from build123d import *

# Parameters (mm, degrees)
SKETCH1_R           = 4
SKETCH1_R_2         = 1.85
BOSS_EXTRUDE1_DEPTH = 3.175


with BuildPart() as part:
    # Sketch1 → Boss-Extrude1 (new body)
    with BuildSketch(Plane.XY):
        with BuildLine():
            Line((-38.1, 100), (38.1, 100))
            Line((38.1, 100), (38.1, 0))
            ThreePointArc((38.1, 0), (0, -38.1), (-38.1, 0))
            Line((-38.1, 0), (-38.1, 100))
        make_face()
        Circle(SKETCH1_R, mode=Mode.SUBTRACT)
        with Locations((-8, 0)):
            Circle(SKETCH1_R_2, mode=Mode.SUBTRACT)
        with Locations((0, -8)):
            Circle(SKETCH1_R_2, mode=Mode.SUBTRACT)
        with Locations((0, 8)):
            Circle(SKETCH1_R_2, mode=Mode.SUBTRACT)
        with Locations((8, 0)):
            Circle(SKETCH1_R_2, mode=Mode.SUBTRACT)
    extrude(amount=BOSS_EXTRUDE1_DEPTH)


solid = part.part
Read the model definition and answer for the solid it produces. Units are mm, in the model's axes. Coordinates: 2 decimals unless noted, no trailing zeros. Loops run counter-clockwise (first coordinate to the right, second up) from the corner with the lowest first, then second, coordinate; pieces in that order, holes last.
Q1. The part is cut by section D-D on x = 16. Write down the section's boundary in (y, z) (3 decimals).
Q2. This flat-tipped pin is pushed along its axis until it touches: pin 1 Ø3 at (x, y) = (29, 57) entering from -Z. Where does it stop, or does it pass through?
Q3. Consider probe 1 along Y at (x, z) = (0, 2.1); probe 2 along Y at (x, z) = (1, 2.9); probe 3 along Y at (x, z) = (-2, 0.75). Determine where each line is inside the solid, lowest interval first.
Q4. The part is cut by section C-C on x = -8. Write down the section's boundary in (y, z) (3 decimals), and give its area (3 significant figures).
Q5. The part is cut by section B-B on z = 1.1. Write down the section's boundary in (x, y), and give its area (3 significant figures).
Q6. The part is cut by section A-A on y = 8. Write down the section's boundary in (x, z) (3 decimals), and give its area (3 significant figures).
Q7. The mould has two halves that part along Y. Classify faces 1 (the face through (38.1, 51, 2)), 2 (the face through (-0.401, 6.194, 1.565)), 3 (the face through (0.84, -38.09, 1.57)): +Y half, -Y half, draft (parallel to the pull), parting line (faces both ways), or undercut.
Results below:
1. outline: (-34.578, 0) - (100, 0) - (100, 3.175) - (-34.578, 3.175) - close
2. pin 1: stops at z = 0
3. probe 1: y = -38.1 to -9.85, -6.15 to -4, 4 to 6.15, 9.85 to 100
3. probe 2: y = -38.09 to -9.56, -6.44 to -3.87, 3.87 to 6.44, 9.56 to 100
3. probe 3: y = -38.05 to -3.46, 3.46 to 100
4. outline: (-37.251, 0) - (-1.85, 0) - (-1.85, 3.175) - (-37.251, 3.175) - close; (1.85, 0) - (100, 0) - (100, 3.175) - (1.85, 3.175) - close
4. area: 424 mm2
5. outline: (-38.1, 0) arc R38.1 ccw to (38.1, 0) - (38.1, 100) - (-38.1, 100) - close; hole circle Ø3.7 at (-8, 0); hole circle Ø8 at (0, 0); hole circle Ø3.7 at (0, -8); hole circle Ø3.7 at (0, 8); hole circle Ø3.7 at (8, 0)
5. area: 9,810 mm2
6. outline: (-38.1, 0) - (-1.85, 0) - (-1.85, 3.175) - (-38.1, 3.175) - close; (1.85, 0) - (38.1, 0) - (38.1, 3.175) - (1.85, 3.175) - close
6. area: 230 mm2
7. face 1: draft
7. face 2: undercut
7. face 3: -Y half
